Read the model definition and answer for the solid it produces. Units are mm, in the model's axes. A direction names the side the tool comes from. Coordinates: 2 decimals unless noted, no trailing zeros. Loops run counter-clockwise (first coordinate to the right, second up) from the corner with the lowest first, then second, coordinate; pieces in that order, holes last. Notation, with made-up numbers: (-6, 62) -> (3, 62) arc R23 ccw to (3, 79) -> close; hole circle Ø2 at (9.25, -8). An arc over 180 degrees is marked (long way). One line per question, with ' | ' between items. Start each with the question number.
```python
from build123d import *

# Parameters (mm, degrees)
CROQUIS1_R                 = 25.465
SALIENTE_EXTRUIR1_DEPTH    = 7.5
CROQUIS2_R                 = 27.965
SALIENTE_EXTRUIR2_DEPTH    = 0.5
SALIENTE_EXTRUIR3_START    = -14.5
CROQUIS2_2_R               = 27.965
SALIENTE_EXTRUIR3_DEPTH    = 0.5
CROQUIS3_R                 = 19
SALIENTE_EXTRUIR4_DEPTH    = 21
CORTAR_EXTRUIR1_DEPTH      = 45.545846608
CORTAR_EXTRUIR1_DEPTH_BACK = 45.545846608
CROQUIS4_R                 = 6
CORTAR_EXTRUIR2_START      = -6
CROQUIS5_R                 = 19
CROQUIS5_R_2               = 12
CORTAR_EXTRUIR2_DEPTH      = 6
TALADRO_ROSCADO_M31_REACH  = 60.109
TALADRO_ROSCADO_M31_BORE_R = 1.25
CROQUIS10_W                = 1.6
CROQUIS10_H                = 12


with BuildPart() as part:
    # Croquis1 → Saliente-Extruir1 (new, symmetric)
    with BuildSketch(Plane(origin=(0, 0, 0), x_dir=(-1, 0, 0), z_dir=(0, 1, 0))):
        with Locations(Location((0, 0, 0), (0, 0, 90))):
            Circle(CROQUIS1_R)
    extrude(amount=SALIENTE_EXTRUIR1_DEPTH, both=True)

    # Croquis2 → Saliente-Extruir2 (add)
    with BuildSketch(Plane(origin=(0, 7.5, 0), x_dir=(-1, 0, 0), z_dir=(0, 1, 0))):
        with Locations(Location((0, 0, 0), (0, 0, 90))):
            Circle(CROQUIS2_R)
    extrude(amount=-SALIENTE_EXTRUIR2_DEPTH)

    # Croquis2<2> → Saliente-Extruir3 (add)
    with BuildSketch(Plane(origin=(0, 7.5, 0), x_dir=(-1, 0, 0), z_dir=(0, 1, 0)).offset(SALIENTE_EXTRUIR3_START)):
        with Locations(Location((0, 0, 0), (0, 0, 90))):
            Circle(CROQUIS2_2_R)
    extrude(amount=-SALIENTE_EXTRUIR3_DEPTH)

    # Croquis3 → Saliente-Extruir4 (add)
    with BuildSketch(Plane(origin=(0, -7.5, 0), x_dir=(-1, 0, 0), z_dir=(0, 1, 0))):
        with Locations(Location((0, 0, 0), (0, 0, 270))):
            Circle(CROQUIS3_R)
    extrude(amount=SALIENTE_EXTRUIR4_DEPTH)

    # Croquis4 → Cortar-Extruir1 (cut, two sides: drawn at the far end of the back side and taken through both)
    with BuildSketch(Plane(origin=(0, -7, 0), x_dir=(-1, 0, 0), z_dir=(0, 1, 0)).offset(-CORTAR_EXTRUIR1_DEPTH_BACK)):
        with Locations(Location((0, 0, 0), (0, 0, 90))):
            Circle(CROQUIS4_R)
    extrude(amount=CORTAR_EXTRUIR1_DEPTH + CORTAR_EXTRUIR1_DEPTH_BACK, mode=Mode.SUBTRACT)

    # Croquis5 → Cortar-Extruir2 (cut)
    with BuildSketch(Plane(origin=(0, 13.5, 0), x_dir=(-1, 0, 0), z_dir=(0, 1, 0)).offset(CORTAR_EXTRUIR2_START)):
        Circle(CROQUIS5_R)
        with Locations(Location((0, 0, 0), (0, 0, 90))):
            Circle(CROQUIS5_R_2, mode=Mode.SUBTRACT)
    extrude(amount=CORTAR_EXTRUIR2_DEPTH, mode=Mode.SUBTRACT)

    # Taladro roscado M31 bore → Taladro roscado M31 (cut, up to next)
    with BuildSketch(Plane(origin=(-12, 0, 12), x_dir=(0, 1, 0), z_dir=(0, 0, 1)), mode=Mode.PRIVATE) as taladro_roscado_m31_sk1:
        with Locations((10.5, -12)):
            Circle(TALADRO_ROSCADO_M31_BORE_R)
    taladro_roscado_m31_tool1 = extrude(taladro_roscado_m31_sk1.sketch, amount=-TALADRO_ROSCADO_M31_REACH, mode=Mode.PRIVATE) & part.part
    add(taladro_roscado_m31_tool1.solids().sort_by_distance((0, 10.5, 12))[0], mode=Mode.SUBTRACT)

    # Croquis10 → Taladro de margen para M32 (revolve, cut)
    with BuildSketch(Plane(origin=(0, 10.5, 0), x_dir=(0, -1, 0), z_dir=(1, 0, 0))):
        with Locations((0.8, 6)):
            Rectangle(CROQUIS10_W, CROQUIS10_H)
    revolve(axis=Axis((0, 10.5, 6.35), (0, 0, -1)), mode=Mode.SUBTRACT)


solid = part.part
```
(1) Section B-B on x = 0 is taken. Write down the section's boundary in (y, z) (3 decimals).
(2) Section A-A on z = 0 is taken. Write down the section's boundary in (x, y) (3 decimals).
(3) Each of these flat-tipped pins is pushed along its axis until it touches: pin 1 Ø2 at (x, y) = (12.5, 1) entering from +Z; pin 2 Ø1.5 at (x, z) = (-4.5, -17) entering from +Y; pin 3 Ø1.5 at (x, y) = (12, 2.5) entering from -Z. Where does it stop, or does it pass through?
(4) Section D-D on y = 4 is taken. Write down the section's boundary in (x, z) (3 decimals), plus the area to 3 significant figures.
(5) Find the intervals of material crossed by probe 1 along Y at (x, z) = (0, -7.75); probe 2 along X at (y, z) = (4.75, 0) (3 decimals); probe 3 along Y at (x, z) = (12, -14), in increasing order. Write a range as from..to.
(6) A tool of negligible diameter and unlimited length cuts with its end or side. For faces 4 (the flat face through (-12, 7.5, -6)), 5 (the cylindrical face through (-15.495, 0.098, -20.208)), 6 (the cylindrical face through (-17.02, -7.25, -22.19)), from which of +Z, -Z, +X, -X, +Y, -Y can it reach the whole face along a straight path? Write none if from no direction.
(7) Section C-C on y = 10.5 is taken. Write down the section's boundary in (x, z), plus the area to 3 significant figures.
(8) Determine the mould class of faces 1 (the cylindrical face through (-17.02, 7.25, -22.19)), 2 (the cylindrical face through (-0.07, 12.1, -8.94)), 3 (the flat face through (-7, -7.5, 0)) for opening direction Y: +Y half, -Y half, draft (parallel to the pull), parting line (faces both ways), or undercut.
Working result:
1) outline: (-7.5, -27.965) -> (-7, -27.965) -> (-7, -25.465) -> (7, -25.465) -> (7, -27.965) -> (7.5, -27.965) -> (7.5, -12) -> (8.9, -12) -> (8.9, -6) -> (-7.5, -6) -> close; (-7.5, 6) -> (9.25, 6) -> (9.25, 12) -> (7.5, 12) -> (7.5, 27.965) -> (7, 27.965) -> (7, 25.465) -> (-7, 25.465) -> (-7, 27.965) -> (-7.5, 27.965) -> close; (11.75, 6) -> (13.5, 6) -> (13.5, 12) -> (11.75, 12) -> close; (12.1, -12) -> (13.5, -12) -> (13.5, -6) -> (12.1, -6) -> close
2) outline: (-27.965, -7.5) -> (-6, -7.5) -> (-6, 13.5) -> (-12, 13.5) -> (-12, 7.5) -> (-27.965, 7.5) -> (-27.965, 7) -> (-25.465, 7) -> (-25.465, -7) -> (-27.965, -7) -> close; (6, -7.5) -> (27.965, -7.5) -> (27.965, -7) -> (25.465, -7) -> (25.465, 7) -> (27.965, 7) -> (27.965, 7.5) -> (12, 7.5) -> (12, 13.5) -> (6, 13.5) -> close
3) pin 1: stops at z = 22.72 | pin 2: stops at y = 7.5 | pin 3: stops at z = -22.85
4) outline: circle Ø50.93 at (0, 0); hole circle Ø12 at (0, 0) | area: 1,920 mm2
5) probe 1: y = -7.5..8.9, 12.1..13.5 | probe 2: x = -25.465..-6, 6..25.465 | probe 3: y = -7.5..7.5
6) face 4: +Y | face 5: none | face 6: +Y, -Y
7) outline: (-1.6, -11.89) -> (-1.6, -5.78) arc R6 cw to (-1.25, 5.87) -> (-1.25, 11.93) arc R12 ccw to start; (1.25, 5.87) arc R6 cw to (1.6, -5.78) -> (1.6, -11.89) arc R12 ccw to (1.25, 11.93) -> close | area: 305 mm2
8) face 1: draft | face 2: undercut | face 3: -Y half
